```python
from build123d import *

# Parameters (mm, degrees)
BOSS_EXTRUDE1_DEPTH              = 5
BOSS_EXTRUDE1_DEPTH_BACK         = 10
SKETCH3_R                        = 24.925
SKETCH3_R_2                      = 1.3
SKETCH6_R                        = 1.65
CUT_EXTRUDE1_DEPTH               = 5
CBORE_FOR_M2_5_SHCS1_D           = 2.5
CBORE_FOR_M2_5_SHCS1_CBORE_D     = 4.5
CBORE_FOR_M2_5_SHCS1_CBORE_DEPTH = 2.5


with BuildPart() as part:
    # Sketch3 → Boss-Extrude1 (new, two sides: drawn at the far end of the back side and taken through both)
    with BuildSketch(Plane(origin=(0, 15, 0), x_dir=(1, 0, 0), z_dir=(0, 1, 0)).offset(-BOSS_EXTRUDE1_DEPTH_BACK)):
        with Locations(Location((-1.2, 0, 0), (0, 0, 180))):
            Circle(SKETCH3_R)
        with Locations(Location((13.8, 0, 0), (0, 0, 180))):
            Circle(SKETCH3_R_2, mode=Mode.SUBTRACT)
        with Locations(Location((3.435254916, -14.265847744, 0), (0, 0, 180))):
            Circle(SKETCH3_R_2, mode=Mode.SUBTRACT)
        with Locations(Location((-13.335254916, -8.816778784, 0), (0, 0, 180))):
            Circle(SKETCH3_R_2, mode=Mode.SUBTRACT)
        with Locations(Location((-13.335254916, 8.816778784, 0), (0, 0, 180))):
            Circle(SKETCH3_R_2, mode=Mode.SUBTRACT)
        with Locations(Location((3.435254916, 14.265847744, 0), (0, 0, 180))):
            Circle(SKETCH3_R_2, mode=Mode.SUBTRACT)
    extrude(amount=BOSS_EXTRUDE1_DEPTH + BOSS_EXTRUDE1_DEPTH_BACK)

    # Sketch6 → Cut-Extrude1 (cut)
    with BuildSketch(Plane.XZ.offset(-5)):
        with Locations((13.8, 0)):
            Circle(SKETCH6_R)
        with Locations((3.435254916, -14.265847744)):
            Circle(SKETCH6_R)
        with Locations((-13.335254915, -8.816778784)):
            Circle(SKETCH6_R)
        with Locations((-13.335254915, 8.816778784)):
            Circle(SKETCH6_R)
        with Locations((3.435254916, 14.265847744)):
            Circle(SKETCH6_R)
    extrude(amount=-CUT_EXTRUDE1_DEPTH, mode=Mode.SUBTRACT)

    # CBORE for M2.5 SHCS1 (through all)
    with Locations(Plane(origin=(0, 20, 0), x_dir=(1, 0, 0), z_dir=(0, 1, 0))):
        with Locations((13.8, 0), (3.435254916, -14.265847744), (-13.335254916, -8.816778784), (3.435254916, 14.265847744), (-13.335254916, 8.816778784)):
            CounterBoreHole(CBORE_FOR_M2_5_SHCS1_D / 2, CBORE_FOR_M2_5_SHCS1_CBORE_D / 2, CBORE_FOR_M2_5_SHCS1_CBORE_DEPTH)


solid = part.part
```
Source: CAD feature listing. Evaluate the final solid. Frame: model axes, mm. A direction names the side the tool comes from. Round coordinates to 2 decimals unless told otherwise and drop trailing zeros. Loops run counter-clockwise (first coordinate to the right, second up) from the corner with the lowest first, then second, coordinate; pieces in that order, holes last.
(1) Section query B-B (x = 13.8). Output: boundary loops of the cut face in (y, z), and give its area (3 significant figures).
From the geometry:
outline: (5, -19.91) - (20, -19.91) - (20, -2.25) - (17.5, -2.25) - (17.5, -1.3) - (10, -1.3) - (10, -1.65) - (5, -1.65) - close; (5, 1.65) - (10, 1.65) - (10, 1.3) - (17.5, 1.3) - (17.5, 2.25) - (20, 2.25) - (20, 19.91) - (5, 19.91) - close
area: 550 mm2
(2) Material intervals for probe 1 along Z at (x, y) = (-13, 8); probe 2 along X at (y, z) = (9.5, -15.5); probe 3 along X at (y, z) = (6.75, -0.5), sorted ascending.
From the geometry:
probe 1: z = -21.95 to -10.43, -7.2 to 7.2, 10.43 to 21.95
probe 2: x = -20.72 to 2.34, 4.53 to 18.32
probe 3: x = -26.12 to 12.23, 15.37 to 23.72
(3) Section query C-C (y = 7.75). Output: boundary loops of the cut face in (x, z) (3 decimals), and give its area (3 significant figures).
From the geometry:
outline: circle Ø49.85 at (-1.2, 0); hole circle Ø3.3 at (-13.335, -8.817); hole circle Ø3.3 at (-13.335, 8.817); hole circle Ø3.3 at (3.435, -14.266); hole circle Ø3.3 at (3.435, 14.266); hole circle Ø3.3 at (13.8, 0)
area: 1,910 mm2
(4) Section query D-D (z = 9.5). Output: boundary loops of the cut face in (x, y), and give its area (3 significant figures).
From the geometry:
outline: (-24.24, 5) - (-14.84, 5) - (-14.84, 10) - (-14.44, 10) - (-14.44, 17.5) - (-15.48, 17.5) - (-15.48, 20) - (-24.24, 20) - close; (-12.23, 10) - (-11.83, 10) - (-11.83, 5) - (21.84, 5) - (21.84, 20) - (-11.19, 20) - (-11.19, 17.5) - (-12.23, 17.5) - close
area: 649 mm2
(5) Pull-direction query (X, two-part tool) for faces 4 (the flat face through (3.4, 17.5, -12.8)), 5 (the flat face through (-1, 20, 0)); classes: +X half, -X half, draft (parallel to the pull), parting line (faces both ways), or undercut.
From the geometry:
face 4: undercut
face 5: draft
(6) Access query for faces 1 (the cylindrical face through (-13.166, 13.698, 10.106)), 2 (the cylindrical face through (15.946, 18.768, -0.676)), 3 (the flat face through (2, 10, 14)). Directions: +Z, -Z, +X, -X, +Y, -Y. A direction counts if a zero-diameter tool reaches every point of the face in a straight line with its end or side. Return the directions, or none.
From the geometry:
face 1: +Y, -Y
face 2: +Y
face 3: -Y
(7) Contact query for flat-ended pins moving along their axis: pin 1 Ø2 at (x, z) = (-13, -8) entering from +Y; pin 2 Ø3 at (x, z) = (3.44, -14.27) entering from -Y; pin 3 Ø6 at (x, y) = (13, 16.5) entering from +Z. Output: stop coordinate, or through.
From the geometry:
pin 1: stops at y = 17.5
pin 2: stops at y = 10
pin 3: stops at z = 22.27
(8) Section query A-A (x = 3). Output: boundary loops of the cut face in (y, z), and give its area (3 significant figures).
From the geometry:
outline: (5, -24.57) - (20, -24.57) - (20, -16.47) - (17.5, -16.47) - (17.5, -15.49) - (10, -15.49) - (10, -15.86) - (5, -15.86) - close; (5, -12.67) - (10, -12.67) - (10, -13.04) - (17.5, -13.04) - (17.5, -12.06) - (20, -12.06) - (20, 12.06) - (17.5, 12.06) - (17.5, 13.04) - (10, 13.04) - (10, 12.67) - (5, 12.67) - close; (5, 15.86) - (10, 15.86) - (10, 15.49) - (17.5, 15.49) - (17.5, 16.47) - (20, 16.47) - (20, 24.57) - (5, 24.57) - close
area: 646 mm2
